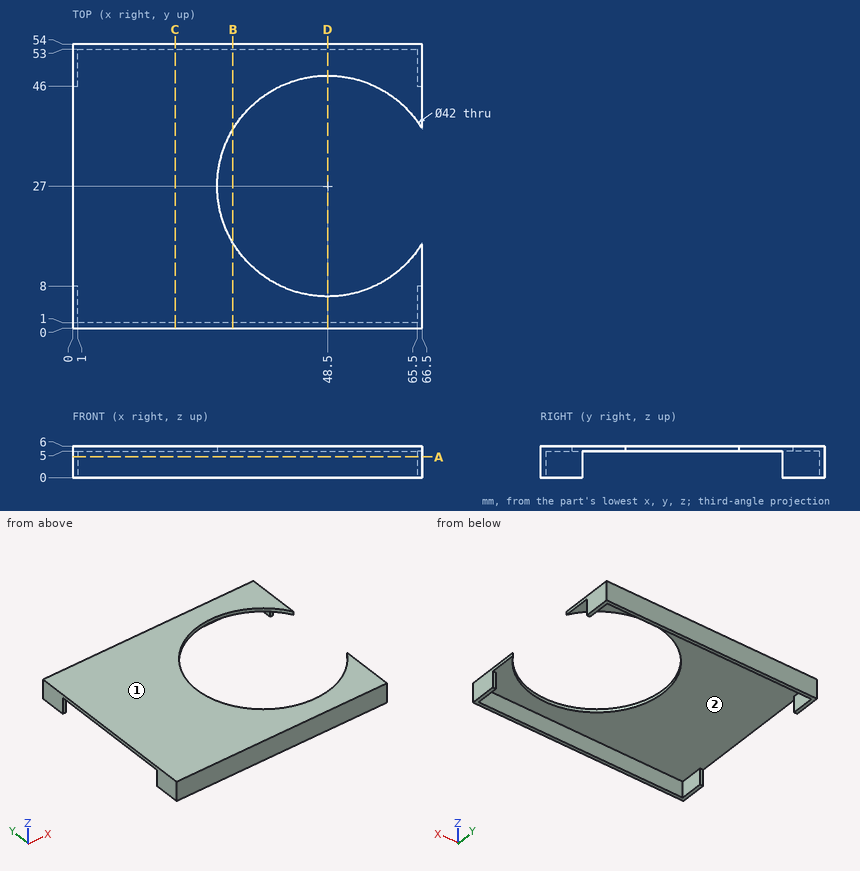
For this review, use the dimensioned drawing (mm, ordinates from the lowest corner) and the shaded views. Round coordinates to 2 decimals unless told otherwise and drop trailing zeros. Order: outer loops, then holes, each group sorted by start corner. A loop starts at its lowest first (then second) coordinate and runs counter-clockwise, first axis right, second up. Notation, with made-up numbers: (-13, 78.5) -> (5, 78.5) arc R25 ccw to (5, 102.5) -> close; hole circle Ø3 at (48, 20.25). An arc over 180 degrees is marked (long way). Put each result on its own line as item: value.
Q1. Add section A-A on z = 3.95. Write out the cut boundary in (x, y).
Check result:
outline: (0, 0) -> (66.5, 0) -> (66.5, 8) -> (65.5, 8) -> (65.5, 1) -> (1, 1) -> (1, 8) -> (0, 8) -> close; (0, 46) -> (1, 46) -> (1, 53) -> (65.5, 53) -> (65.5, 46) -> (66.5, 46) -> (66.5, 54) -> (0, 54) -> close
Q2. Mouldability with a two-part tool opening along X and no side actions: class the marked faces 1 and 2 as pulls with the +X half, pulls with the -X half, needs draft (parallel to the pull), parting line crosses it, or undercut.
Check result:
face 1: needs draft
face 2: undercut
Q3. For probe 1 along Y at (x, z) = (48.5, 5.55); probe 2 along X at (y, z) = (3.5, 3); probe 3 along Y at (x, z) = (50, 4), list the stretches that pass through material, from the lowest coordinate up. Write a range as [from, to].
Check result:
probe 1: [0, 6], [48, 54]
probe 2: [0, 1], [65.5, 66.5]
probe 3: [0, 1], [53, 54]
Q4. Add section B-B on x = 30.5. Write out the cut boundary in (y, z), plus the area to 3 significant figures.
Check result:
outline: (0, 0) -> (1, 0) -> (1, 5) -> (16.18, 5) -> (16.18, 6) -> (0, 6) -> close; (37.82, 5) -> (53, 5) -> (53, 0) -> (54, 0) -> (54, 6) -> (37.82, 6) -> close
area: 42.4 mm2
Q5. Add section D-D on x = 48.5. Write out the cut boundary in (y, z).
Check result:
outline: (0, 0) -> (1, 0) -> (1, 5) -> (6, 5) -> (6, 6) -> (0, 6) -> close; (48, 5) -> (53, 5) -> (53, 0) -> (54, 0) -> (54, 6) -> (48, 6) -> close
Q6. Add section C-C on x = 19.5. Write out the cut boundary in (y, z), plus the area to 3 significant figures.
Check result:
outline: (0, 0) -> (1, 0) -> (1, 5) -> (53, 5) -> (53, 0) -> (54, 0) -> (54, 6) -> (0, 6) -> close
area: 64.0 mm2
